```python
from build123d import *

# Parameters (mm, degrees)
BOSS_EXTRUDE1_DEPTH            = 1.6
F_3_5_3_5_DIAMETER_HOLE1_D     = 3.5
F_3_5_3_5_DIAMETER_HOLE1_DEPTH = 3
F_3_5_3_5_DIAMETER_HOLE1_TIP   = 1.051506083


with BuildPart() as part:
    # Sketch2 → Boss-Extrude1 (new body)
    with BuildSketch(Plane(origin=(0, 0, 0), x_dir=(1, 0, 0), z_dir=(0, 1, 0))):
        Polygon((50.8, -22.47), (50.8, 11.586871141), (48.2, 14.186871141), (48.2, 24.07), (45.6, 26.67), (-50.8, 26.67), (-50.8, -26.67), (48.2, -26.67), (48.2, -25.07), align=None)
    extrude(amount=BOSS_EXTRUDE1_DEPTH)

    # Ø3.5 (3.5) Diameter Hole1
    with Locations(Plane(origin=(0, 1.6, 0), x_dir=(-1, 0, 0), z_dir=(0, 1, 0))):
        with Locations((35.468438844, -24.132254762), (35.468438844, 23.898881858), (-45.502928223, 23.898881858), (-39.195511542, -24.132254762)):
            Hole(F_3_5_3_5_DIAMETER_HOLE1_D / 2, depth=F_3_5_3_5_DIAMETER_HOLE1_DEPTH)
            with Locations((0, 0, -(F_3_5_3_5_DIAMETER_HOLE1_DEPTH + F_3_5_3_5_DIAMETER_HOLE1_TIP / 2))):  # 118° drill point
                Cone(0, F_3_5_3_5_DIAMETER_HOLE1_D / 2, F_3_5_3_5_DIAMETER_HOLE1_TIP, mode=Mode.SUBTRACT)


solid = part.part
```
CAD build for the part. Positions are in the model's coordinates, mm. Coordinates: 2 decimals unless noted, no trailing zeros. Write each loop counter-clockwise with the first axis right and the second up, starting at its lowest first coordinate (ties: lowest second). Pieces come first, ordered by that corner, then holes. Notation, with made-up numbers: (52, 35.5) -> (87, 35.5) arc R26 ccw to (87, 52.5) -> close; hole circle Ø5 at (82.5, 56). An arc over 180 degrees is marked (long way). Return JSON: item names as keys, results as strings. Group by question number.
Q1. Pull direction X, two halves, no side cores. Call faces 1 (the face through (49.518, 0.789, -12.869)), 2 (the face through (40.14, 0.79, -22.66)), 3 (the face through (-33.85, 0.79, 23.23)), 4 (the face through (-1, 0, 0)): released by +X, released by -X, zero draft, split by the parting line, or undercut.
Q2. Cut at B-B, the plane y = 1.3. Give the cut face in (x, z), then the cut area to 3 significant figures.
Q3. Flat gauge pin, fed straight in: pin 1 (0.8 mm diameter, centred on y = 0.5, z = -21.5, fed in from +X). Where does the tip first touch, or does it go through?
Q4. Cut at A-A, the plane x = 39. Give the cut face in (y, z), then the cut area to 3 significant figures.
Q5. Drill centre lines: line 1 (X direction, y = 0.3, z = 24); line 2 (X direction, y = 0.5, z = -17.5); line 3 (X direction, y = 0.95, z = -12). Where is each one in solid material? Low to high.
Returned:
{
 "1": {"face 1": "released by +X", "face 2": "undercut", "face 3": "undercut", "face 4": "zero draft"},
 "2": {"outline": "(-50.8, -26.67) -> (45.6, -26.67) -> (48.2, -24.07) -> (48.2, -14.19) -> (50.8, -11.59) -> (50.8, 22.47) -> (48.2, 25.07) -> (48.2, 26.67) -> (-50.8, 26.67) -> close; hole circle Ø3.5 at (-35.47, -24.13); hole circle Ø3.5 at (-35.47, 23.9); hole circle Ø3.5 at (39.2, -24.13); hole circle Ø3.5 at (45.5, 23.9)", "area": "5,330 mm2"},
 "3": {"pin 1": "stops at x = 48.2"},
 "4": {"outline": "(0, -26.67) -> (1.6, -26.67) -> (1.6, -25.87) -> (0, -25.87) -> close; (0, -22.39) -> (1.6, -22.39) -> (1.6, 26.67) -> (0, 26.67) -> close", "area": "79.8 mm2"},
 "5": {"line 1": "x = -50.8 to -37.22, -33.72 to 43.76, 47.25 to 49.27", "line 2": "x = -50.8 to 48.2", "line 3": "x = -50.8 to 50.39"}
}
